Build history of the part. All positions in model axes, mm. A direction names the side the tool comes from. Give positions to 0.01 mm unless a question says otherwise; leave off trailing zeros. Order: outer loops, then holes, each group sorted by start corner. A loop starts at its lowest first (then second) coordinate and runs counter-clockwise, first axis right, second up. Notation, with made-up numbers: M 1.25,36.25 L 31.25,36.25 A9 cw 31.25,52.25 Z; hole C 32.25,-17 d1. An arc over 180 degrees is marked long. One line per item, written item: value.
Autodesk Inventor part; units mm, degrees
ref_plane "YZ Plane" through (0, 0, 0) normal (1, 0, 0) x (0, 1, 0)
ref_plane "XZ Plane" through (0, 0, 0) normal (0, 1, 0) x (-1, 0, 0)
ref_plane "XY Plane" through (0, 0, 0) normal (0, 0, 1) x (1, 0, 0)
sketch "スケッチ1" plane through (0, 0, 0) normal (0, 1, 0) x (-1, 0, 0)
  line L0 (-20, 45) -> (20, 45)
  line L1 (20, 45) -> (20, -45)
  line L2 (20, -45) -> (-20, -45)
  line L3 (-20, -45) -> (-20, 45)
  line L4 (-20, 45) -> (20, -45) construction
  line L5 (20, 45) -> (-20, -45) construction
  point P0 (0, 0)
  dimension "d0" = 90
  dimension "d1" = 40
extrude "プレート1" add sketch "スケッチ1" along normal blind 2.3
sketch "スケッチ2" plane through (17.7, 2.3, 45) normal (1, 0, 0) x (0, 1, 0)
  line L0 (0, -90) -> (0, 0)
  line L1 (0, 0) -> (-12.6, 0)
  line L2 (-12.6, 0) -> (-12.6, -90)
  line L3 (-12.6, -90) -> (0, -90)
edge flange "フランジ1" height 12.6 angle 90 thickness 2.3 bend radius 2.3 thickness toward (1, 0, 0) relief tear relief width 2.3 relief depth 1.15 edges at (20, 0, 0) wall of the first edge with corners at (17.7, 2.3, -45) (17.7, 2.3, 45) (17.7, -10.3, 45) (17.7, -10.3, -45)
bend "曲げ1"
corner "コーナー1"
sketch "スケッチ3" plane through (-17.7, 0, 45) normal (-1, 0, 0) x (0, -1, 0)
  line L0 (0, -90) -> (0, 0)
  line L1 (0, 0) -> (-30, 0)
  line L2 (-30, 0) -> (-30, -90)
  line L3 (-30, -90) -> (0, -90)
edge flange "フランジ2" height 30 angle 90 thickness 2.3 bend radius 2.3 thickness toward (-1, 0, 0) relief tear relief width 2.3 relief depth 1.15 edges at (-20, 2.3, 0) wall of the first edge with corners at (-17.7, 0, -45) (-17.7, 0, 45) (-17.7, 30, 45) (-17.7, 30, -45)
bend "曲げ2"
corner "コーナー2"
sketch "スケッチ4" plane through (20, -10.3, 45) normal (1, 0, 0) x (0, 0, -1)
  line L0 (90, 0) -> (0, 0)
  line L1 (0, 0) -> (0, 8)
  point P0 (45, 10.3)
  point P1 (5, 4)
  point P2 (85, 4)
  dimension "d23" = 4
  dimension "d24" = 80
  dimension "d25" = 5
hole "穴1" at (20, -6.3, 40) at (20, -6.3, -40) direction (-1, 0, 0) diameter 3.2 depth 2.3 tip angle 118
fillet "コーナーR1" radius 4 4 edges at (18.85, -10.3, 45) (18.85, -10.3, -45) (-18.85, 30, -45) (-18.85, 30, 45)
equation "\"d31\" = Thickness"
equation "\"d2\" = Thickness"
equation "\"d3\" = BendReliefWidth"
equation "\"d4\" = BendReliefDepth"
equation "\"d5\" = MinimumRemnant"
equation "\"d6\" = TransitionRadius"
equation "\"d9\" = BendRadius"
equation "\"d10\" = CornerReliefSize"
equation "\"d11\" = GapSize"
equation "\"d12\" = JacobiRadiusSize"
equation "\"d13\" = BendReliefWidth"
equation "\"d14\" = BendReliefDepth"
equation "\"d15\" = MinimumRemnant"
equation "\"d16\" = TransitionRadius"
equation "\"d19\" = BendRadius"
equation "\"d20\" = CornerReliefSize"
equation "\"d21\" = GapSize"
equation "\"d22\" = JacobiRadiusSize"
equation "\"BendRadius\" = Thickness"
equation "\"BendReliefWidth\" = Thickness"
equation "\"BendReliefDepth\" = 0.5 * Thickness"
equation "\"CornerReliefSize\" = 4 * Thickness"
equation "\"MinimumRemnant\" = 2 * Thickness"
equation "\"TransitionRadius\" = BendRadius"
equation "\"JacobiRadiusSize\" = BendRadius"
equation "\"GapSize\" = Thickness"
properties part number "plate7" material "鋼、炭素鋼"
1) Saw through at D-D, the plane y = 22.5. Write the cut outline in (x, z).
Check values:
outline: M -20,-45 L -17.7,-45 L -17.7,45 L -20,45 Z
2) Saw through at A-A, the plane z = -40. Write the cut outline in (x, y).
Check values:
outline: M -20,4.6 A4.6 ccw -15.4,0 L 15.4,0 A2.3 cw 17.7,-2.3 L 17.7,-4.7 L 20,-4.7 L 20,-2.3 A4.6 ccw 15.4,2.3 L -15.4,2.3 A2.3 cw -17.7,4.6 L -17.7,30 L -20,30 Z; M 17.7,-10.3 L 20,-10.3 L 20,-7.9 L 17.7,-7.9 Z
3) Drill centre lines: probe 1 along Z at (x, y) = (19.55, -6.3); probe 2 along Y at (x, z) = (4, -16.5); probe 3 along X at (y, z) = (7, -24). Where is each one in solid material? Low to high. Write a range as from..to.
Check values:
probe 1: -45..-41.6, -38.4..38.4, 41.6..45
probe 2: 0..2.3
probe 3: -20..-17.7
4) Tool access for faces 4 (the face through (-17.7, 17, 1)), 5 (the face through (17.7, -6, 1)), 6 (the face through (-8, 2, -45)): list every direction of +Z, -Z, +X, -X, +Y, -Y with a clear straight run to the whole face (end or side of a thin tool).
Check values:
face 4: +Z, -Z, +X, +Y
face 5: +Z, -Z, -X, -Y
face 6: -Z, +X, -X, +Y, -Y
5) Pin check, flat tips, straight feed: pin 1 (2.5 mm diameter, centred on y = -6.3, z = -40, fed in from -X); pin 2 (3 mm diameter, centred on x = -8, z = -29, fed in from +Y); pin 3 (4 mm diameter, centred on y = -7.5, z = 11.5, fed in from -X); pin 4 (2 mm diameter, centred on x = -5.5, z = 22.5, fed in from -Y). Stop position of each tip, or through.
Check values:
pin 1: through
pin 2: y = 2.3
pin 3: x = 17.7
pin 4: y = 0
6) Saw through at B-B, the plane z = -13. Write the cut outline in (x, y), then the cut area to 3 significant figures.
Check values:
outline: M -20,4.6 A4.6 ccw -15.4,0 L 15.4,0 A2.3 cw 17.7,-2.3 L 17.7,-10.3 L 20,-10.3 L 20,-2.3 A4.6 ccw 15.4,2.3 L -15.4,2.3 A2.3 cw -17.7,4.6 L -17.7,30 L -20,30 Z
area: 173 mm^2
7) Saw through at C-C, the plane x = 8. Write the cut outline in (y, z).
Check values:
outline: M 0,-45 L 2.3,-45 L 2.3,45 L 0,45 Z
8) Mould opens along Z. For faces 1 (the face through (-17.04, 2.99, 0.63)), 2 (the face through (18.83, -4.74, -39.65)), 3 (the face through (-18.866, 28.797, 43.859)) say: released by +Z, released by -Z, zero draft, split by the parting line, or undercut.
Check values:
face 1: zero draft
face 2: undercut
face 3: released by +Z
